```python
from build123d import *

# Parameters (mm, degrees)
SKETCH1_W           = 130
SKETCH1_H           = 18
BOSS_EXTRUDE1_DEPTH = 4
SKETCH2_W           = 4
SKETCH2_H           = 5
CUT_EXTRUDE1_DEPTH  = 66.741919656
SKETCH3_R           = 1.5
CUT_EXTRUDE2_DEPTH  = 66.741919656
SKETCH4_R           = 1.5
CUT_EXTRUDE3_DEPTH  = 66.741919656


with BuildPart() as part:
    # Sketch1 → Boss-Extrude1 (new body)
    with BuildSketch(Plane(origin=(0, 0, 0), x_dir=(1, 0, 0), z_dir=(0, 1, 0))):
        Rectangle(SKETCH1_W, SKETCH1_H)
    extrude(amount=BOSS_EXTRUDE1_DEPTH)

    # Sketch2 → Cut-Extrude1 (cut, through all)
    with BuildSketch(Plane(origin=(0, 4, 0), x_dir=(1, 0, 0), z_dir=(0, 1, 0))):
        with Locations((57, -4.5)):
            Rectangle(SKETCH2_W, SKETCH2_H)
        with Locations((57, 4.5)):
            Rectangle(SKETCH2_W, SKETCH2_H)
        with Locations((-57, -4.5)):
            Rectangle(SKETCH2_W, SKETCH2_H)
        with Locations((-57, 4.5)):
            Rectangle(SKETCH2_W, SKETCH2_H)
        with Locations((48, -4.5)):
            Rectangle(SKETCH2_W, SKETCH2_H)
        with Locations((48, 4.5)):
            Rectangle(SKETCH2_W, SKETCH2_H)
        with Locations((39, -4.5)):
            Rectangle(SKETCH2_W, SKETCH2_H)
        with Locations((39, 4.5)):
            Rectangle(SKETCH2_W, SKETCH2_H)
        with Locations((30, -4.5)):
            Rectangle(SKETCH2_W, SKETCH2_H)
        with Locations((30, 4.5)):
            Rectangle(SKETCH2_W, SKETCH2_H)
        with Locations((-48, 4.5)):
            Rectangle(SKETCH2_W, SKETCH2_H)
        with Locations((-30, 4.5)):
            Rectangle(SKETCH2_W, SKETCH2_H)
        with Locations((-30, -4.5)):
            Rectangle(SKETCH2_W, SKETCH2_H)
        with Locations((-39, 4.5)):
            Rectangle(SKETCH2_W, SKETCH2_H)
        with Locations((-39, -4.5)):
            Rectangle(SKETCH2_W, SKETCH2_H)
        with Locations((-48, -4.5)):
            Rectangle(SKETCH2_W, SKETCH2_H)
    extrude(amount=-CUT_EXTRUDE1_DEPTH, mode=Mode.SUBTRACT)

    # Sketch3 → Cut-Extrude2 (cut, through all)
    with BuildSketch(Plane.XZ):
        with Locations(Location((17, -0.95, 0), (0, 0, 270))):
            Circle(SKETCH3_R)
        with Locations(Location((-10, -0.95, 0), (0, 0, 270))):
            Circle(SKETCH3_R)
        with Locations(Location((-17, -0.95, 0), (0, 0, 270))):
            Circle(SKETCH3_R)
        with Locations(Location((10, -0.95, 0), (0, 0, 270))):
            Circle(SKETCH3_R)
    extrude(amount=-CUT_EXTRUDE2_DEPTH, mode=Mode.SUBTRACT)

    # Sketch4 → Cut-Extrude3 (cut, through all)
    with BuildSketch(Plane(origin=(0, 4, 0), x_dir=(1, 0, 0), z_dir=(0, 1, 0))):
        with Locations(Location((4, 0.45, 0), (0, 0, 270))):
            Circle(SKETCH4_R)
        with Locations(Location((-4, 0.45, 0), (0, 0, 270))):
            Circle(SKETCH4_R)
        with Locations((-20, -7.55)):
            Circle(SKETCH4_R)
        with Locations((20, -7.55)):
            Circle(SKETCH4_R)
    extrude(amount=-CUT_EXTRUDE3_DEPTH, mode=Mode.SUBTRACT)


solid = part.part
```
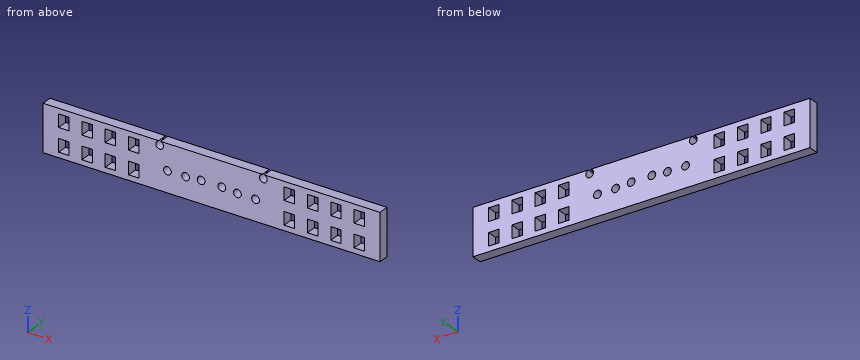
Input: part model. Units: mm. Frame: model coordinates. Coordinates: 2 decimals unless noted, no trailing zeros. Write each loop counter-clockwise with the first axis right and the second up, starting at its lowest first coordinate (ties: lowest second). Pieces come first, ordered by that corner, then holes.
1) Material intervals for line 1 along Z through (x, y) = (-58, 1.6); line 2 along X through (y, z) = (2.9, 7.55); line 3 along Z through (x, y) = (-20, 2.85), sorted ascending.
2) Section C-C on y = 1.5. State how many separate pieces and enclosed holes the cut face has, and give its area (3 significant figures).
3) Section A-A on x = -29.5. Output: boundary loops of the cut face in (y, z), and give its area (3 significant figures).
4) Section B-B on x = -4. Output: boundary loops of the cut face in (y, z), and give its area (3 significant figures).
Check result:
1. line 1: z = -9 to -7, -2 to 2, 7 to 9
1. line 2: x = -65 to -21.5, -18.5 to 18.5, 21.5 to 65
1. line 3: z = -9 to 6.05
2. separate pieces: 1
2. enclosed holes: 22
2. area: 1,960 mm2
3. outline: (0, -9) - (4, -9) - (4, -7) - (0, -7) - close; (0, -2) - (4, -2) - (4, 2) - (0, 2) - close; (0, 7) - (4, 7) - (4, 9) - (0, 9) - close
3. area: 32.0 mm2
4. outline: (0, -9) - (4, -9) - (4, -1.95) - (0, -1.95) - close; (0, 1.05) - (4, 1.05) - (4, 9) - (0, 9) - close
4. area: 60.0 mm2
